The model under review builds one solid part; all positions refer to its coordinate system, in mm. A direction names the side the tool comes from. Give positions to 0.01 mm unless a question says otherwise; leave off trailing zeros. Order: outer loops, then holes, each group sorted by start corner. A loop starts at its lowest first (then second) coordinate and runs counter-clockwise, first axis right, second up. Notation, with made-up numbers: (42, -13) - (101, -13) arc R21 cw to (101, 16) - close; hole circle Ø7 at (-31.75, 4.5). An arc over 180 degrees is marked (long way). Write item = value, one per line. Start each with the question number.
1. Mouldability with a two-part tool opening along X and no side actions: class faces 4 (the flat face through (-37.919, -68, -1)), 5 (the flat face through (-13, -132.7, -1)), 6 (the flat face through (9, -6, -1)) as pulls with the +X half, pulls with the -X half, needs draft (parallel to the pull), parting line crosses it, or undercut.
2. Wall thickness on probe 1 along Y at (x, z) = (13, -2); probe 2 along Y at (x, z) = (29, -1.9): over which ranges is each line inside the solid? List them lowest first.
3. We need section B-B, the plane x = -30.5. Give the boundary of the cut face in (y, z).
4. For P1, Ø0.9, axis at x = 9.5, z = -1, coming from the +Y side; P2, Ø1, axis at x = -27, y = -115.5, coming from the +Z side; P3, Ø0.9, axis at y = -4.5, z = -2, coming from the +X side; P4, Ø1.5, axis at y = -4, z = -1.5, coming from the -X side, all flat-tipped, find the tip position at first contact; note any pin that passes through.
5. We need section C-C, the plane x = -9.5. Give the boundary of the cut face in (y, z), and give its area (3 significant figures).
6. Machinability: for faces 1 (the flat face through (-25.369, -4, -1)), 2 (the flat face through (-11.269, -4, -1)), 3 (the flat face through (9, -128, -1)), which of the approach directions +Z, -Z, +X, -X, +Y, -Y give a long, thin tool a straight path to every point of the face, cutting with its end or side? Answer none if there is none.
7. We need section A-A, the plane z = -1.75. Give the boundary of the cut face in (x, y).
Autodesk Inventor part; units mm, degrees
ref_plane "YZ Plane" through (0, 0, 0) normal (1, 0, 0) x (0, 1, 0)
ref_plane "XZ Plane" through (0, 0, 0) normal (0, 1, 0) x (-1, 0, 0)
ref_plane "XY Plane" through (0, 0, 0) normal (0, 0, 1) x (1, 0, 0)
sketch "NewProfile" plane through (0, 0, 0) normal (0, 0, 1) x (1, 0, 0)
  line L0 (28.6811, -6) -> (28.8811, -4)
  line L1 (44.2811, -6) -> (28.6811, -6)
  line L2 (44.0811, -4) -> (44.2811, -6)
  line L3 (28.8811, -4) -> (44.0811, -4)
  line L4 (-10.7189, -4) -> (-10.5189, -6)
  line L5 (-25.9189, -4) -> (-10.7189, -4)
  line L6 (-26.1189, -6) -> (-25.9189, -4)
  line L7 (-10.5189, -6) -> (-26.1189, -6)
  line L8 (44.2811, -128) -> (44.0811, -130)
  line L9 (28.6811, -128) -> (44.2811, -128)
  line L10 (28.8811, -130) -> (28.6811, -128)
  line L11 (44.0811, -130) -> (28.8811, -130)
  line L12 (-26.1189, -128) -> (-25.9189, -130)
  line L13 (-10.7189, -130) -> (-25.9189, -130)
  line L14 (-10.5189, -128) -> (-10.7189, -130)
  line L15 (-26.1189, -128) -> (-10.5189, -128)
  line L16 (-37.9189, -6) -> (56.0811, -6)
  line L17 (56.0811, -6) -> (56.0811, -128)
  line L18 (56.0811, -128) -> (-37.9189, -128)
  line L19 (-37.9189, -128) -> (-37.9189, -6)
  line L20 (-25.3689, -6) -> (-11.2689, -6)
  line L21 (-11.2689, -6) -> (-11.2689, -1.3)
  line L22 (-11.2689, -1.3) -> (-25.3689, -1.3)
  line L23 (-25.3689, -1.3) -> (-25.3689, -6)
  line L24 (29.4311, -6) -> (43.5311, -6)
  line L25 (43.5311, -6) -> (43.5311, -1.3)
  line L26 (43.5311, -1.3) -> (29.4311, -1.3)
  line L27 (29.4311, -1.3) -> (29.4311, -6)
  line L28 (-26.1189, -128) -> (-26.1189, -6) construction
  line L29 (-21.1189, -128) -> (-20.9189, -130) construction
  line L30 (-5.7189, -130) -> (-20.9189, -130) construction
  line L31 (-5.7189, -130) -> (-5.5189, -128) construction
  line L32 (-21.1189, -128) -> (-5.5189, -128) construction
  line L33 (39.0811, -130) -> (39.2811, -128) construction
  line L34 (23.6811, -128) -> (39.2811, -128) construction
  line L35 (23.8811, -130) -> (23.6811, -128) construction
  line L36 (39.0811, -130) -> (23.8811, -130) construction
  line L37 (-21.1189, -128) -> (-21.1189, -6) construction
  line L38 (-21.1189, -128) -> (100.8811, -128) construction
  line L39 (-10.5189, -128) -> (-10.5189, -6) construction
  line L40 (-10.5189, -128) -> (111.4811, -128) construction
  line L41 (-5.5189, -128) -> (-5.5189, -6) construction
  line L42 (-5.5189, -128) -> (116.4811, -128) construction
  line L43 (23.6811, -128) -> (23.6811, -6) construction
  line L44 (28.6811, -128) -> (28.6811, -6) construction
  line L45 (39.2811, -128) -> (39.2811, -6) construction
  line L46 (44.2811, -128) -> (44.2811, -6) construction
  line L47 (-5.5189, -6) -> (-5.7189, -4) construction
  line L48 (-20.9189, -4) -> (-5.7189, -4) construction
  line L49 (-20.9189, -4) -> (-21.1189, -6) construction
  line L50 (-5.5189, -6) -> (-21.1189, -6) construction
  line L51 (39.2811, -6) -> (39.0811, -4) construction
  line L52 (23.8811, -4) -> (39.0811, -4) construction
  line L53 (23.8811, -4) -> (23.6811, -6) construction
  line L54 (39.2811, -6) -> (23.6811, -6) construction
  line L55 (-20.5689, -128) -> (-6.4689, -128)
  line L56 (-6.4689, -128) -> (-6.4689, -132.7)
  line L57 (-6.4689, -132.7) -> (-20.5689, -132.7)
  line L58 (-20.5689, -132.7) -> (-20.5689, -128)
  line L59 (24.2311, -128) -> (38.3311, -128)
  line L60 (38.3311, -128) -> (38.3311, -132.7)
  line L61 (38.3311, -132.7) -> (24.2311, -132.7)
  line L62 (24.2311, -132.7) -> (24.2311, -128)
  point P0 (0, 0)
  dimension "d0" = 94
  dimension "d1" = 122
  dimension "d2" = 11.8
  dimension "d3" = 11.8
  dimension "d4" = 14.1
  dimension "d5" = 4.7
  dimension "d6" = 14.1
  dimension "d7" = 4.7
  dimension "d21" = 0.55
  dimension "d23" = 15.2
  dimension "d24" = 15.2
  dimension "d25" = 0.55
  dimension "d26" = 14.1
  dimension "d27" = 4.7
  dimension "d28" = 14.1
  dimension "d29" = 4.7
  dimension "d30" = 15.2
  dimension "d31" = 0.55
  dimension "d32" = 0.55
  dimension "d33" = 15.2
extrude "Extrusion1" add sketch "NewProfile" against normal blind 3 contours L1 L16 L17 L18 L9 L15 L19 L7 | L27 L3 L25 L1 | L27 L26 L25 L3 | L7 L23 L5 L21 | L5 L23 L22 L21 | L60 L11 L10 L9 | L60 L61 L62 L18 L10 L11 | L15 L14 L13 L58 | L13 L14 L18 L56 L57 L58
equation "\"d21\" = -0.5 * d4 + 0.5 * d23"
equation "\"d25\" = -0.5 * d6 + 0.5 * d24"
equation "\"d31\" = -0.5 * d26 + 0.5 * d30"
equation "\"d32\" = -0.5 * d28 + 0.5 * d33"
properties part number "SideWall_new"
Model answer:
q1.face_4 = pulls with the -X half
q1.face_5 = needs draft
q1.face_6 = undercut
q2.probe_1 = -128 to -6
q2.probe_2 = -132.7 to -6
q3.outline = (-128, -3) - (-6, -3) - (-6, 0) - (-128, 0) - close
q4.P1 = -6
q4.P2 = 0
q4.P3 = 43.53
q4.P4 = -25.37
q5.outline = (-132.7, -3) - (-6, -3) - (-6, 0) - (-132.7, 0) - close
q5.area = 380 mm2
q6.face_1 = +Z, -Z, -X, +Y
q6.face_2 = +Z, -Z, +Y
q6.face_3 = +Z, -Z, -Y
q7.outline = (-37.92, -128) - (-20.57, -128) - (-20.57, -132.7) - (-6.47, -132.7) - (-6.47, -128) - (24.23, -128) - (24.23, -132.7) - (38.33, -132.7) - (38.33, -128) - (56.08, -128) - (56.08, -6) - (43.53, -6) - (43.53, -1.3) - (29.43, -1.3) - (29.43, -6) - (-11.27, -6) - (-11.27, -1.3) - (-25.37, -1.3) - (-25.37, -6) - (-37.92, -6) - close
